from build123d import *

# Parameters (mm, degrees)
SKETCH1_R           = 5
SKETCH1_R_2         = 2.45
BOSS_EXTRUDE1_DEPTH = 8
SKETCH2_R           = 10
SKETCH2_R_2         = 3.95
CUT_EXTRUDE1_DEPTH  = 4
CHAMFER1_SIZE       = 0.3


with BuildPart() as part:
    # Sketch1 → Boss-Extrude1 (new body)
    with BuildSketch(Plane(origin=(0, 0, 0), x_dir=(1, 0, 0), z_dir=(0, 1, 0))):
        with Locations(Location((0, 0, 0), (0, 0, 270))):
            Circle(SKETCH1_R)
        with Locations(Location((0, 0, 0), (0, 0, 270))):
            Circle(SKETCH1_R_2, mode=Mode.SUBTRACT)
    extrude(amount=BOSS_EXTRUDE1_DEPTH)

    # Sketch2 → Cut-Extrude1 (cut)
    with BuildSketch(Plane(origin=(0, 8, 0), x_dir=(1, 0, 0), z_dir=(0, 1, 0))):
        Circle(SKETCH2_R)
        with Locations(Location((0, 0, 0), (0, 0, 270))):
            Circle(SKETCH2_R_2, mode=Mode.SUBTRACT)
    extrude(amount=-CUT_EXTRUDE1_DEPTH, mode=Mode.SUBTRACT)

    # Chamfer1
    chamfer1_edges = [part.edges().sort_by_distance(p)[0] for p in [
        (0, 8, -3.95),
        (0, 4, -5),
        (0, 0, -5),
        (0, 0, -2.45),
        (0, 8, -2.45),
    ]]
    chamfer(chamfer1_edges, length=CHAMFER1_SIZE)


solid = part.part
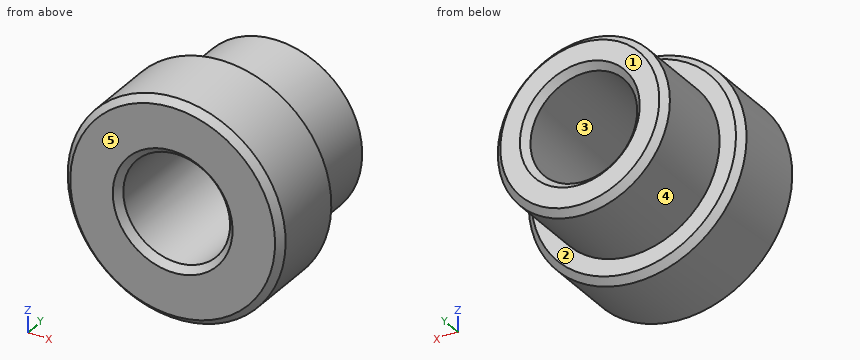
Design review of the part built by this model. Coordinates are the model's own, in mm. Face numbers are marked on the shaded views. A direction names the side the tool comes from. Round coordinates to 2 decimals unless told otherwise and drop trailing zeros. Write each loop counter-clockwise with the first axis right and the second up, starting at its lowest first coordinate (ties: lowest second). Pieces come first, ordered by that corner, then holes.
Item 1: Consider section B-B on z = 0. Give the boundary of the cut face in (x, y).
Item 2: Draft analysis for pull direction X (two halves, no side actions). For the marked faces 3, 4 and 5, state which applies: released by +X, released by -X, zero draft, split by the parting line, or undercut.
Item 3: Consider section D-D on y = 0.75. Give the boundary of the cut face in (x, z).
Item 4: Wall thickness on L1, parallel to X at y = 2.5, z = 0; L2, parallel to X at y = 5.5, z = 0; L3, parallel to Y at x = 4, z = 2.25: over which ranges is each line inside the solid? List them lowest first.
Item 5: For pin 1 Ø3 at (x, y) = (3, 6.5) entering from +Z; pin 2 Ø4.5 at (x, z) = (0, 0) entering from -Y; pin 3 Ø1 at (x, z) = (3, 3.5) entering from +Y; pin 4 Ø3 at (x, y) = (2, 2) entering from +Z, all flat-tipped, find the tip position at first contact; note any pin that passes through.
Item 6: Consider section A-A on x = 0. Give the boundary of the cut face in (y, z).
Item 7: Consider section C-C on y = 6.25. Give the boundary of the cut face in (x, z).
Item 8: For the marked faces 1 and 2, list the 3-axis set-ups (+Z, -Z, +X, -X, +Y, -Y) from which the entire face can be reached by the end or side of a thin tool; tool diameter is ignored.
Check values:
1. outline: (-5, 0.3) - (-4.7, 0) - (-2.75, 0) - (-2.45, 0.3) - (-2.45, 7.7) - (-2.75, 8) - (-3.65, 8) - (-3.95, 7.7) - (-3.95, 4) - (-4.7, 4) - (-5, 3.7) - close; (2.45, 0.3) - (2.75, 0) - (4.7, 0) - (5, 0.3) - (5, 3.7) - (4.7, 4) - (3.95, 4) - (3.95, 7.7) - (3.65, 8) - (2.75, 8) - (2.45, 7.7) - close
2. face 3: undercut
2. face 4: split by the parting line
2. face 5: zero draft
3. outline: circle Ø10 at (0, 0); hole circle Ø4.9 at (0, 0)
4. L1: x = -5 to -2.45, 2.45 to 5
4. L2: x = -3.95 to -2.45, 2.45 to 3.95
4. L3: y = 0 to 4
5. pin 1: stops at z = 3.65
5. pin 2: passes through
5. pin 3: stops at y = 4
5. pin 4: stops at z = 4.97
6. outline: (0, -4.7) - (0.3, -5) - (3.7, -5) - (4, -4.7) - (4, -3.95) - (7.7, -3.95) - (8, -3.65) - (8, -2.75) - (7.7, -2.45) - (0.3, -2.45) - (0, -2.75) - close; (0, 2.75) - (0.3, 2.45) - (7.7, 2.45) - (8, 2.75) - (8, 3.65) - (7.7, 3.95) - (4, 3.95) - (4, 4.7) - (3.7, 5) - (0.3, 5) - (0, 4.7) - close
7. outline: circle Ø7.9 at (0, 0); hole circle Ø4.9 at (0, 0)
8. face 1: +Z, -Z, +X, -X, +Y
8. face 2: +Y
